Autodesk Inventor part; units mm, degrees
ref_plane "YZ Plane" through (0, 0, 0) normal (1, 0, 0) x (0, 1, 0)
ref_plane "XZ Plane" through (0, 0, 0) normal (0, 1, 0) x (-1, 0, 0)
ref_plane "XY Plane" through (0, 0, 0) normal (0, 0, 1) x (1, 0, 0)
sketch "スケッチ1" plane through (0, 0, 0) normal (0, 0, 1) x (1, 0, 0)
  arc A0 (-23.45, 0) -> (23.45, 0) centre (0, 0) ccw
  arc A1 (-36.55, 0) -> (36.55, 0) centre (0, 0) ccw
  circle A2 centre (0, -30) radius 2.55
  circle A3 centre (28.1908, -10.2606) radius 2.55
  circle A4 centre (-28.1908, -10.2606) radius 2.55
  line L0 (0, 0) -> (-28.1908, -10.2606) construction
  line L1 (0, 0) -> (28.1908, -10.2606) construction
  line L2 (-48.309, 0) -> (65.7551, 0)
  dimension "d0" = 46.9
  dimension "d1" = 73.1
  dimension "d2" = 5.1
  dimension "d3" = 5.1
  dimension "d4" = 5.1
  dimension "d5" = 30
  dimension "d6" = 30
  dimension "d7" = 30
  dimension "d9" = 20
  dimension "d10" = 20
extrude "押し出し1" add sketch "スケッチ1" along normal blind 10 contours A0 L2 A1
fillet "フィレット1" radius 2 4 edges at (36.55, 0, 5) (23.45, 0, 5) (-23.45, 0, 5) (-36.55, 0, 5)
sketch "スケッチ3" plane through (0, 0, 10) normal (0, 0, 1) x (1, 0, 0)
  circle A0 centre (0, 0) radius 23.45
  circle A1 centre (0, 0) radius 36.55
  circle A2 centre (28.1908, -10.2606) radius 2.55
  circle A3 centre (28.1908, -10.2606) radius 2.55
  circle A4 centre (0, -30) radius 2.55
  circle A5 centre (0, -30) radius 2.55
  circle A6 centre (-28.1908, -10.2606) radius 2.55
  circle A7 centre (-28.1908, -10.2606) radius 2.55
extrude "押し出し3" add sketch "スケッチ3" against normal blind 10
sketch "スケッチ5" plane through (0, 0, 10) normal (0, 0, 1) x (1, 0, 0)
  circle A0 centre (-28.1908, -10.2606) radius 2.55
  circle A1 centre (-28.1908, -10.2606) radius 3
  circle A2 centre (0, -30) radius 2.55
  circle A3 centre (0, -30) radius 3
  circle A4 centre (28.1908, -10.2606) radius 2.55
  circle A5 centre (28.1908, -10.2606) radius 3
  point P0 (0, 0)
  dimension "d22" = 6
  dimension "d23" = 6
  dimension "d24" = 6
extrude "押し出し5" cut sketch "スケッチ5" against normal through all
properties part number "半円 穴あり"
Build history of the part. All positions in model axes, mm. Give positions to 0.01 mm unless a question says otherwise; leave off trailing zeros. Loops run counter-clockwise (first coordinate to the right, second up) from the corner with the lowest first, then second, coordinate; pieces in that order, holes last. Notation, with made-up numbers: (81.5, 47) -> (87.5, 47) arc R24 ccw to (87.5, 84) -> close; hole circle Ø4 at (55.5, -20). An arc over 180 degrees is marked (long way). Answer in a Markdown table with one row per item.
Item 1: Probe line 1 along Y through (x, z) = (0, 4.25); line 2 along Y through (x, z) = (1, 3.25); line 3 along X through (y, z) = (0, 6.25). List the from-to ranges inside material, lowest first. Write a range as [from, to].
Findings below:
| item | result |
|---|---|
| line 1 | y = [-36.55, -33], [-27, -23.45], [23.45, 36.55] |
| line 2 | y = [-36.54, -32.83], [-27.17, -23.43], [23.43, 36.54] |
| line 3 | x = [-36.55, -23.45], [23.45, 36.55] |
Item 2: Mould opens along Y. For faces 1 (the flat face through (24, 1, 10)), 2 (the cylindrical face through (-7.92, -35.68, 5.07)), 3 (the cylindrical face through (22.37, 7.04, 5.07)) say: pulls with the +Y half, pulls with the -Y half, needs draft (parallel to the pull), parting line crosses it, or undercut.
Findings below:
| item | result |
|---|---|
| face 1 | needs draft |
| face 2 | parting line crosses it |
| face 3 | undercut |
Item 3: Slice it at D-D on y = -12. Write the cut outline in (x, z).
Findings below:
| item | result |
|---|---|
| outline | (-34.52, 0) -> (-30.64, 0) -> (-30.64, 10) -> (-34.52, 10) -> close; (-25.75, 0) -> (-20.15, 0) -> (-20.15, 10) -> (-25.75, 10) -> close; (20.15, 0) -> (25.75, 0) -> (25.75, 10) -> (20.15, 10) -> close; (30.64, 0) -> (34.52, 0) -> (34.52, 10) -> (30.64, 10) -> close |
Item 4: Slice it at C-C on x = -22.5. Write the cut outline in (y, z).
Findings below:
| item | result |
|---|---|
| outline | (-28.8, 0) -> (-6.61, 0) -> (-6.61, 10) -> (-28.8, 10) -> close; (6.61, 0) -> (28.8, 0) -> (28.8, 10) -> (6.61, 10) -> close |
Item 5: Slice it at A-A on y = 0. Write the cut outline in (x, z).
Findings below:
| item | result |
|---|---|
| outline | (-36.55, 0) -> (-23.45, 0) -> (-23.45, 10) -> (-36.55, 10) -> close; (23.45, 0) -> (36.55, 0) -> (36.55, 10) -> (23.45, 10) -> close |
Item 6: Slice it at B-B on x = 0. Write the cut outline in (y, z).
Findings below:
| item | result |
|---|---|
| outline | (-36.55, 0) -> (-33, 0) -> (-33, 10) -> (-36.55, 10) -> close; (-27, 0) -> (-23.45, 0) -> (-23.45, 10) -> (-27, 10) -> close; (23.45, 0) -> (36.55, 0) -> (36.55, 10) -> (23.45, 10) -> close |
Item 7: Flat gauge pins, fed straight in: P1, Ø3, axis at y = -6, z = 9, coming from the -X side; P2, Ø1.5, axis at x = -10.5, z = 3.5, coming from the -Y side; P3, Ø4, axis at x = -11, z = 7, coming from the +Y side. Where does each tip first touch, or does it go through?
Findings below:
| item | result |
|---|---|
| P1 | stops at x = -36.27 |
| P2 | stops at y = -35.23 |
| P3 | stops at y = 35.42 |
